The model under review builds one solid part; all positions refer to its coordinate system, in mm. Round coordinates to 2 decimals unless told otherwise and drop trailing zeros. Order: outer loops, then holes, each group sorted by start corner. A loop starts at its lowest first (then second) coordinate and runs counter-clockwise, first axis right, second up. Notation, with made-up numbers: M 17,-39.75 L 23,-39.75 A26 ccw 23,-3.75 Z; hole C -34.5,-35 d4. An arc over 180 degrees is marked long. Answer as a JSON object with one key per item and string values. Group by question number.
1) Consider section C-C, the plane y = 5.25. Count the separate pieces of the cut face and the enclosed holes in it, then the cut area to 3 significant figures.
2) Consider section B-B, the plane x = 1.4. Write out the cut boundary in (y, z), then the cut area to 3 significant figures.
3) Consider section D-D, the plane x = 6.75. Write out the cut boundary in (y, z).
4) Consider section A-A, the plane z = -8.6. Write out the cut boundary in (x, y), then the cut area to 3 significant figures.
5) Insertion check: pin 1 Ø0.9 at (x, z) = (8.5, -1.5) entering from +Y. The pin has a flat end and moves straight along its axis. Give the tip position at first contact, or say it passes through.
6) To check wall thickness, follow line 1 (X direction, y = 5.5, z = -1.4); line 2 (Z direction, x = 8.6, y = 5.5); line 3 (Z direction, x = 5, y = 5). State the ranges of each line that lie inside material, in increasing order.
```python
from build123d import *

# Parameters (mm, degrees)
SKETCH1_W               = 10
SKETCH1_H               = 10
BOSS_EXTRUDE1_DEPTH     = 6.35
FILLET1_R               = 1
SKETCH2_R               = 0.4
CUT_EXTRUDE1_DEPTH      = 1.6
LPATTERN1_COUNT         = 5
LPATTERN1_PITCH         = 1.808
LPATTERN2_COUNT         = 5
LPATTERN2_PITCH         = 1.808
MIRROR2_COPY_1_SKETCH_R = 0.4
MIRROR2_COPY_1_DEPTH    = 1.6
MIRROR2_COPY_2_SKETCH_R = 0.4
MIRROR2_COPY_2_DEPTH    = 1.6
MIRROR2_COPY_3_SKETCH_R = 0.4
MIRROR2_COPY_3_DEPTH    = 1.6
MIRROR2_COPY_4_SKETCH_R = 0.4
MIRROR2_COPY_4_DEPTH    = 1.6
MIRROR3_COPY_1_SKETCH_R = 0.4
MIRROR3_COPY_1_DEPTH    = 1.6
MIRROR3_COPY_2_SKETCH_R = 0.4
MIRROR3_COPY_2_DEPTH    = 1.6
MIRROR3_COPY_3_SKETCH_R = 0.4
MIRROR3_COPY_3_DEPTH    = 1.6
MIRROR3_COPY_4_SKETCH_R = 0.4
MIRROR3_COPY_4_DEPTH    = 1.6


with BuildPart() as part:
    # Sketch1 → Boss-Extrude1 (new body)
    with BuildSketch(Plane(origin=(0, 0, 0), x_dir=(1, 0, 0), z_dir=(0, 1, 0))):
        with Locations((5, 5)):
            Rectangle(SKETCH1_W, SKETCH1_H)
    extrude(amount=BOSS_EXTRUDE1_DEPTH)

    # Fillet1
    fillet1_edges = [part.edges().sort_by_distance(p)[0] for p in [
        (0, 3.175, -10),
        (10, 3.175, -10),
        (10, 3.175, 0),
        (0, 3.175, 0),
    ]]
    fillet(fillet1_edges, radius=FILLET1_R)

    # Sketch2 → Cut-Extrude1 (cut)
    with BuildSketch(Plane(origin=(0, 6.35, 0), x_dir=(1, 0, 0), z_dir=(0, 1, 0))):
        with Locations((1.4, 8.6)):
            Circle(SKETCH2_R)
    cut_extrude1 = extrude(amount=-CUT_EXTRUDE1_DEPTH, mode=Mode.SUBTRACT)

    # LPattern1: Cut-Extrude1 ×5
    with Locations(*[(i * LPATTERN1_PITCH, 0, 0) for i in range(1, LPATTERN1_COUNT)]):
        add(cut_extrude1, mode=Mode.SUBTRACT)

    # LPattern2: Cut-Extrude1 ×5
    with Locations(*[(0, 0, i * LPATTERN2_PITCH) for i in range(1, LPATTERN2_COUNT)]):
        add(cut_extrude1, mode=Mode.SUBTRACT)

    # Mirror2: Cut-Extrude1 across plane
    add(cut_extrude1.mirror(Plane.ZY.offset(-5)), mode=Mode.SUBTRACT)

    # Mirror2 copy 1 sketch → Mirror2 copy 1 (cut)
    with BuildSketch(Plane(origin=(10, 6.35, 1.808), x_dir=(-1, 0, 0), z_dir=(0, 1, 0))):
        with Locations((1.4, -8.6)):
            Circle(MIRROR2_COPY_1_SKETCH_R)
    extrude(amount=-MIRROR2_COPY_1_DEPTH, mode=Mode.SUBTRACT)

    # Mirror2 copy 2 sketch → Mirror2 copy 2 (cut)
    with BuildSketch(Plane(origin=(10, 6.35, 3.616), x_dir=(-1, 0, 0), z_dir=(0, 1, 0))):
        with Locations((1.4, -8.6)):
            Circle(MIRROR2_COPY_2_SKETCH_R)
    extrude(amount=-MIRROR2_COPY_2_DEPTH, mode=Mode.SUBTRACT)

    # Mirror2 copy 3 sketch → Mirror2 copy 3 (cut)
    with BuildSketch(Plane(origin=(10, 6.35, 5.424), x_dir=(-1, 0, 0), z_dir=(0, 1, 0))):
        with Locations((1.4, -8.6)):
            Circle(MIRROR2_COPY_3_SKETCH_R)
    extrude(amount=-MIRROR2_COPY_3_DEPTH, mode=Mode.SUBTRACT)

    # Mirror2 copy 4 sketch → Mirror2 copy 4 (cut)
    with BuildSketch(Plane(origin=(10, 6.35, 7.232), x_dir=(-1, 0, 0), z_dir=(0, 1, 0))):
        with Locations((1.4, -8.6)):
            Circle(MIRROR2_COPY_4_SKETCH_R)
    extrude(amount=-MIRROR2_COPY_4_DEPTH, mode=Mode.SUBTRACT)

    # Mirror3: Cut-Extrude1 across plane
    add(cut_extrude1.mirror(Plane(origin=(0, 0, -5), x_dir=(1, 0, 0), z_dir=(0, 0, -1))), mode=Mode.SUBTRACT)

    # Mirror3 copy 1 sketch → Mirror3 copy 1 (cut)
    with BuildSketch(Plane(origin=(1.808, 6.35, -10), x_dir=(1, 0, 0), z_dir=(0, 1, 0))):
        with Locations((1.4, -8.6)):
            Circle(MIRROR3_COPY_1_SKETCH_R)
    extrude(amount=-MIRROR3_COPY_1_DEPTH, mode=Mode.SUBTRACT)

    # Mirror3 copy 2 sketch → Mirror3 copy 2 (cut)
    with BuildSketch(Plane(origin=(3.616, 6.35, -10), x_dir=(1, 0, 0), z_dir=(0, 1, 0))):
        with Locations((1.4, -8.6)):
            Circle(MIRROR3_COPY_2_SKETCH_R)
    extrude(amount=-MIRROR3_COPY_2_DEPTH, mode=Mode.SUBTRACT)

    # Mirror3 copy 3 sketch → Mirror3 copy 3 (cut)
    with BuildSketch(Plane(origin=(5.424, 6.35, -10), x_dir=(1, 0, 0), z_dir=(0, 1, 0))):
        with Locations((1.4, -8.6)):
            Circle(MIRROR3_COPY_3_SKETCH_R)
    extrude(amount=-MIRROR3_COPY_3_DEPTH, mode=Mode.SUBTRACT)

    # Mirror3 copy 4 sketch → Mirror3 copy 4 (cut)
    with BuildSketch(Plane(origin=(7.232, 6.35, -10), x_dir=(1, 0, 0), z_dir=(0, 1, 0))):
        with Locations((1.4, -8.6)):
            Circle(MIRROR3_COPY_4_SKETCH_R)
    extrude(amount=-MIRROR3_COPY_4_DEPTH, mode=Mode.SUBTRACT)


solid = part.part
```
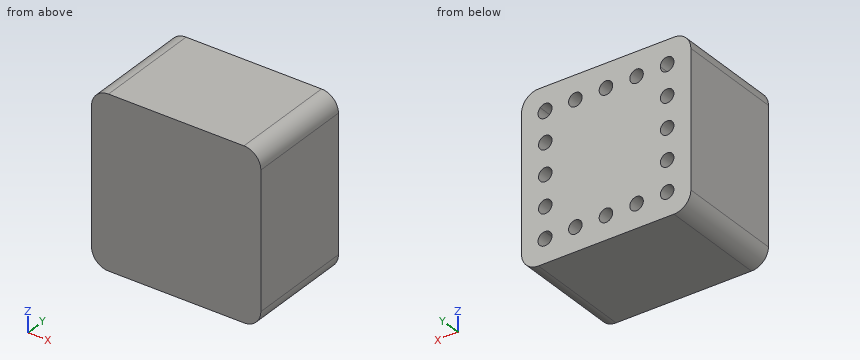
Results list:
{
 "1": {"separate pieces": "1", "enclosed holes": "16", "area": "91.0 mm^2"},
 "2": {"outline": "M 0,-10 L 6.35,-10 L 6.35,-9 L 4.75,-9 L 4.75,-8.2 L 6.35,-8.2 L 6.35,-7.19 L 4.75,-7.19 L 4.75,-6.39 L 6.35,-6.39 L 6.35,-5.38 L 4.75,-5.38 L 4.75,-4.58 L 6.35,-4.58 L 6.35,-3.58 L 4.75,-3.58 L 4.75,-2.78 L 6.35,-2.78 L 6.35,-1.8 L 4.75,-1.8 L 4.75,-0.97 L 6.35,-0.97 L 6.35,0 L 0,0 Z", "area": "57.0 mm^2"},
 "3": {"outline": "M 0,-10 L 6.35,-10 L 6.35,-8.99 L 4.75,-8.99 L 4.75,-8.21 L 6.35,-8.21 L 6.35,-1.79 L 4.75,-1.79 L 4.75,-1.01 L 6.35,-1.01 L 6.35,0 L 0,0 Z"},
 "4": {"outline": "M 0,0 L 10,0 L 10,6.35 L 9.03,6.35 L 9.03,4.75 L 8.2,4.75 L 8.2,6.35 L 7.22,6.35 L 7.22,4.75 L 6.42,4.75 L 6.42,6.35 L 5.42,6.35 L 5.42,4.75 L 4.62,4.75 L 4.62,6.35 L 3.61,6.35 L 3.61,4.75 L 2.81,4.75 L 2.81,6.35 L 1.8,6.35 L 1.8,4.75 L 1,4.75 L 1,6.35 L 0,6.35 Z", "area": "57.0 mm^2"},
 "5": {"pin 1": "y = 6.35"},
 "6": {"line 1": "0 to 1, 1.8 to 2.81, 3.61 to 4.62, 5.42 to 6.42, 7.22 to 8.2, 9.03 to 10", "line 2": "-10 to -9, -8.2 to -7.19, -6.39 to -5.38, -4.58 to -3.58, -2.78 to -1.8, -0.97 to 0", "line 3": "-10 to -9, -8.2 to -1.8, -1 to 0"}
}
